The model under review builds one solid part; all positions refer to its coordinate system, in mm. A direction names the side the tool comes from. Round coordinates to 2 decimals unless told otherwise and drop trailing zeros. Loops run counter-clockwise (first coordinate to the right, second up) from the corner with the lowest first, then second, coordinate; pieces in that order, holes last. Notation, with made-up numbers: (4.5, 3.25) -> (28.5, 3.25) arc R23 cw to (28.5, 32.25) -> close; hole circle Ø11 at (-34.75, -37.75). An arc over 180 degrees is marked (long way). Write each question's results on one line, items separated by ' | '. Start each with the question number.
Item 1: We need section A-A (x = 0). Give the boundary of the cut face in (y, z), and give its area (3 significant figures).
Item 2: We need section B-B (z = -8). Give the boundary of the cut face in (x, y).
Item 3: We need section D-D (x = -4). Give the boundary of the cut face in (y, z).
Item 4: Clearance check with flat-ended pins moving along their axes: pin 1 Ø5 at (x, y) = (13, -7) entering from -Z; pin 2 Ø2 at (x, z) = (6, 8) entering from -Y; pin 3 Ø5 at (x, z) = (-15, -5.5) entering from -Y. State where each tip first meets the part, or that it passes through.
Item 5: Tool access review of faces 5 (the flat face through (0, 0, 0)), 6 (the flat face through (13.9, 3.683, -4.6)), 7 (the flat face through (-6, 0, 10)): name each direction out of +Z, -Z, +X, -X, +Y, -Y from which nothing blocks a thin tool from reaching the whole face with its end or side.
Item 6: For L1, parallel to X at y = 7.5, z = -6; L2, parallel to X at y = 0.25, z = 7; L3, parallel to X at y = 5, z = -6.75, list the stretches that pass through material, from the lowest coordinate up. Write a range as from..to.
Item 7: Mouldability with a two-part tool opening along X and no side actions: class faces 1 (the flat face through (-14, 6, -11.938)), 2 (the cylindrical face through (-14.894, 6.187, -5.523)), 3 (the cylindrical face through (12.606, 6.187, -5.523)), 4 (the flat face through (16.256, 1.8, 0.2)) as pulls with the +X half, pulls with the -X half, needs draft (parallel to the pull), parting line crosses it, or undercut.
Item 8: We need section C-C (y = -5.25). Give the boundary of the cut face in (x, z), and give its area (3 significant figures).
from build123d import *

# Parameters (mm, degrees)
SKETCH1_W                   = 32.512
SKETCH1_H                   = 17.526
BOSS_EXTRUDE1_DEPTH         = 5.08
SKETCH2_W                   = 4.758
SKETCH2_H                   = 5.08
SKETCH2_W_2                 = 4.746
BOSS_EXTRUDE2_DEPTH         = 11.938
F_40_0_098_DIAMETER_HOLE1_D = 2.4892
BOSS_EXTRUDE3_DEPTH         = 10.16
F_6_0_204_DIAMETER_HOLE2_D  = 5.1816


with BuildPart() as part:
    # Sketch1 → Boss-Extrude1 (new body)
    with BuildSketch(Plane.XY):
        Rectangle(SKETCH1_W, SKETCH1_H)
    extrude(amount=BOSS_EXTRUDE1_DEPTH)

    # Sketch2 → Boss-Extrude2 (add)
    with BuildSketch(Plane(origin=(0, 0, 0), x_dir=(-1, 0, 0), z_dir=(0, 0, -1))):
        with Locations((13.877, 6.223)):
            Rectangle(SKETCH2_W, SKETCH2_H)
        with Locations((-13.883, 6.223)):
            Rectangle(SKETCH2_W_2, SKETCH2_H)
    extrude(amount=BOSS_EXTRUDE2_DEPTH)

    # #40 (0.098) Diameter Hole1 (through all)
    with Locations(Plane(origin=(0, 8.763, 0), x_dir=(1, 0, 0), z_dir=(0, 1, 0))):
        with Locations((-13.744, 6), (13.756, 6)):
            Hole(F_40_0_098_DIAMETER_HOLE1_D / 2)

    # Sketch5 → Boss-Extrude3 (add)
    with BuildSketch(Plane.XY.offset(5.08)):
        with BuildLine():
            Line((7.62, 0), (4.953, 0))
            ThreePointArc((4.953, 0), (0, 4.953), (-4.953, 0))
            Line((-4.953, 0), (-7.62, 0))
            ThreePointArc((-7.62, 0), (0, 7.62), (7.62, 0))
        make_face()
    extrude(amount=BOSS_EXTRUDE3_DEPTH)

    # #6 (0.204) Diameter Hole2 (through all)
    with Locations(Plane(origin=(0, 7.62, 0), x_dir=(1, 0, 0), z_dir=(0, 1, 0))):
        with Locations((0, -10.16)):
            Hole(F_6_0_204_DIAMETER_HOLE2_D / 2)


solid = part.part
Here are the results:
1) outline: (-8.76, 0) -> (8.76, 0) -> (8.76, 5.08) -> (7.62, 5.08) -> (7.62, 7.57) -> (4.95, 7.57) -> (4.95, 5.08) -> (-8.76, 5.08) -> close; (4.95, 12.75) -> (7.62, 12.75) -> (7.62, 15.24) -> (4.95, 15.24) -> close | area: 102 mm2
2) outline: (-16.26, 3.68) -> (-11.5, 3.68) -> (-11.5, 8.76) -> (-16.26, 8.76) -> close; (11.51, 3.68) -> (16.26, 3.68) -> (16.26, 8.76) -> (11.51, 8.76) -> close
3) outline: (-8.76, 0) -> (8.76, 0) -> (8.76, 5.08) -> (6.49, 5.08) -> (6.49, 15.24) -> (2.92, 15.24) -> (2.92, 5.08) -> (-8.76, 5.08) -> close
4) pin 1: stops at z = 0 | pin 2: stops at y = 0 | pin 3: stops at y = 3.68
5) face 5: -Z, -Y | face 6: -Z, +X, -X, -Y | face 7: +Z, +X, -X, -Y
6) L1: x = -16.26..-14.99, -12.5..-11.5, 11.51..12.51, 15..16.26 | L2: x = -7.62..-4.95, 4.95..7.62 | L3: x = -16.26..-14.74, -12.75..-11.5, 11.51..12.76, 14.75..16.26
7) face 1: needs draft | face 2: undercut | face 3: undercut | face 4: pulls with the +X half
8) outline: (-16.26, 0) -> (16.26, 0) -> (16.26, 5.08) -> (-16.26, 5.08) -> close | area: 165 mm2
